Model file for the job. Use its own axes, mm. Round coordinates to 2 decimals unless told otherwise and drop trailing zeros. Order: outer loops, then holes, each group sorted by start corner. A loop starts at its lowest first (then second) coordinate and runs counter-clockwise, first axis right, second up. Notation, with made-up numbers: (29, 18) - (68, 18) arc R32 ccw to (68, 45) - close; hole circle Ø1 at (44.25, 62). An arc over 180 degrees is marked (long way). Use one line per item in the form item = value.
from build123d import *

# Parameters (mm, degrees)
CROQUIS1_R              = 4.5
CROQUIS1_R_2            = 2.5
SALIENTE_EXTRUIR1_DEPTH = 11
CHAFL_N1_SIZE           = 0.5


# Read off the part's stored shape, not the designer's step: Cortar-Barrer1
with BuildPart() as part:
    # Croquis1 → Saliente-Extruir1 (new body)
    with BuildSketch(Plane.XY):
        Circle(CROQUIS1_R)
        Circle(CROQUIS1_R_2, mode=Mode.SUBTRACT)
    extrude(amount=SALIENTE_EXTRUIR1_DEPTH)

    # Chaflán1
    chafl_n1_edges = [part.edges().sort_by_distance(p)[0] for p in [
        (-4.5, 0, 0),
        (-4.5, 0, 11),
    ]]
    chamfer(chafl_n1_edges, length=CHAFL_N1_SIZE)

    # Cortar-Barrer1 outline → Cortar-Barrer1 (revolve, cut)
    with BuildSketch(Plane.XZ):
        with BuildLine():
            Line((4.5, 6.4387505), (4.5, 9.5612495))
            ThreePointArc((4.5, 9.5612495), (3.75, 8), (4.5, 6.4387505))
        make_face()
    revolve(axis=Axis((0, 0, 0), (0, 0, 1)), mode=Mode.SUBTRACT)


solid = part.part
(1) Slice it at D-D on z = 9. Give the cut face in (x, y), then the cut area to 3 significant figures.
Report:
outline = circle Ø8.04 at (0, 0); hole circle Ø5 at (0, 0)
area = 31.1 mm2
(2) Probe probe 1 along Y at (x, z) = (2, 6.25); probe 2 along Z at (x, y) = (1.5, 4). List the from-to ranges inside material, lowest first. Write a range as [from, to].
Report:
probe_1 = [-4.03, -1.5], [1.5, 4.03]
probe_2 = [0.27, 6.65], [9.35, 10.73]
(3) Slice it at C-C on z = 5.5. Give the cut face in (x, y).
Report:
outline = circle Ø9 at (0, 0); hole circle Ø5 at (0, 0)
(4) Pull direction X, two halves, no side cores. Call faces 1 (the face through (-0.54, -2.44, 5.42)), 2 (the face through (-0.59, 4.46, 10.02)), 3 (the face through (-2, -2, 11)): released by +X, released by -X, zero draft, split by the parting line, or undercut.
Report:
face_1 = undercut
face_2 = split by the parting line
face_3 = zero draft
(5) Slice it at A-A on y = 0. Give the cut face in (x, z).
Report:
outline = (-4.5, 0.5) - (-4, 0) - (-2.5, 0) - (-2.5, 11) - (-4, 11) - (-4.5, 10.5) - (-4.5, 9.56) arc R2 cw to (-4.5, 6.44) - close; (2.5, 0) - (4, 0) - (4.5, 0.5) - (4.5, 6.44) arc R2 cw to (4.5, 9.56) - (4.5, 10.5) - (4, 11) - (2.5, 11) - close
(6) Pin check, flat tips, straight feed: pin 1 (1.5 mm diameter, centred on y = 2.5, z = 2.5, fed in from +X); pin 2 (5 mm diameter, centred on x = 1.5, z = 10, fed in from +Y); pin 3 (4 mm diameter, centred on x = -2, z = 8, fed in from -Y). Stop position of each tip, or through.
Report:
pin_1 = 4.15
pin_2 = 4.5
pin_3 = -4.44
